```python
from build123d import *

# Parameters (mm, degrees)
SKETCH2_R               = 2.1828125
BOSS_EXTRUDE1_DEPTH     = 3.175
SKETCH3_W               = 36.843225838
SKETCH3_H               = 9.525
BOSS_EXTRUDE2_DEPTH     = 25.4
SKETCH4_R               = 2.1828125
SKETCH4_W               = 0.959112919
SKETCH4_H               = 25.4
SKETCH4_W_2             = 15.875
SKETCH4_H_2             = 15.875
CUT_EXTRUDE1_DEPTH      = 1
CUT_EXTRUDE1_DEPTH_BACK = 10.525
FILLET1_R               = 1.5875
CHAMFER1_SIZE           = 0.396875


with BuildPart() as part:
    # Sketch2 → Boss-Extrude1 (new body)
    with BuildSketch(Plane(origin=(0, 0, 0), x_dir=(1, 0, 0), z_dir=(0, 1, 0))):
        with BuildLine():
            Line((-38.1, 4.7625), (38.1, 4.7625))
            ThreePointArc((38.1, 4.7625), (42.8625, 0), (38.1, -4.7625))
            Line((38.1, -4.7625), (-38.1, -4.7625))
            ThreePointArc((-38.1, -4.7625), (-42.8625, 0), (-38.1, 4.7625))
        make_face()
        with Locations((-38.1, 0)):
            Circle(SKETCH2_R, mode=Mode.SUBTRACT)
        with Locations((38.1, 0)):
            Circle(SKETCH2_R, mode=Mode.SUBTRACT)
    extrude(amount=BOSS_EXTRUDE1_DEPTH)

    # Sketch3 → Boss-Extrude2 (add)
    with BuildSketch(Plane(origin=(0, 3.175, 0), x_dir=(1, 0, 0), z_dir=(0, 1, 0))):
        Rectangle(SKETCH3_W, SKETCH3_H)
    extrude(amount=BOSS_EXTRUDE2_DEPTH)

    # Sketch4 → Cut-Extrude1 (cut, two sides)
    with BuildSketch(Plane.XY.offset(4.7625)) as cut_extrude1_sk:
        with Locations((-12.7, 23.8125)):
            Circle(SKETCH4_R)
        with Locations((12.7, 23.8125)):
            Circle(SKETCH4_R)
        with Locations((-17.94205646, 15.875)):
            Rectangle(SKETCH4_W, SKETCH4_H)
        with Locations((17.94205646, 15.875)):
            Rectangle(SKETCH4_W, SKETCH4_H)
        with Locations((0, 11.1125)):
            Rectangle(SKETCH4_W_2, SKETCH4_H_2)
    extrude(amount=CUT_EXTRUDE1_DEPTH, mode=Mode.SUBTRACT)
    extrude(cut_extrude1_sk.sketch, amount=-CUT_EXTRUDE1_DEPTH_BACK, mode=Mode.SUBTRACT)

    # Fillet1
    fillet1_edges = [part.edges().sort_by_distance(p)[0] for p in [
        (-17.4625, 3.175, 0),
        (-17.4625, 28.575, 0),
        (17.4625, 28.575, 0),
        (17.4625, 3.175, 0),
        (-7.9375, 3.175, 0),
        (-7.9375, 19.05, 0),
        (7.9375, 19.05, 0),
        (7.9375, 3.175, 0),
    ]]
    fillet(fillet1_edges, radius=FILLET1_R)

    # Chamfer1
    chamfer1_edges = [part.edges().sort_by_distance(p)[0] for p in [
        (0, 28.575, -4.7625),
        (0, 28.575, 4.7625),
        (0, 3.175, 4.7625),
        (-7.9375, 11.1125, 4.7625),
        (0, 19.05, 4.7625),
        (7.9375, 11.1125, 4.7625),
        (-17.4625, 15.875, 4.7625),
        (28.575, 3.175, 4.7625),
        (17.4625, 15.875, 4.7625),
        (16.997532015, 28.110032015, 4.7625),
        (-16.997532015, 28.110032015, 4.7625),
        (-17.4625, 15.875, -4.7625),
        (0, 19.05, -4.7625),
        (-7.9375, 11.1125, -4.7625),
        (0, 3.175, -4.7625),
        (7.9375, 11.1125, -4.7625),
        (-28.575, 3.175, -4.7625),
        (17.4625, 15.875, -4.7625),
        (16.997532015, 28.110032015, -4.7625),
        (-16.997532015, 28.110032015, -4.7625),
        (-40.2828125, 0, 0),
        (-17.927467985, 3.639967985, 4.7625),
        (-40.2828125, 3.175, 0),
        (-17.927467985, 3.639967985, -4.7625),
        (17.927467985, 3.639967985, 4.7625),
        (17.927467985, 3.639967985, -4.7625),
        (-7.472532015, 18.585032015, 4.7625),
        (42.8625, 3.175, 0),
        (-7.472532015, 18.585032015, -4.7625),
        (7.472532015, 18.585032015, 4.7625),
        (7.472532015, 18.585032015, -4.7625),
        (7.472532015, 3.639967985, 4.7625),
        (7.472532015, 3.639967985, -4.7625),
        (-7.472532015, 3.639967985, 4.7625),
        (-7.472532015, 3.639967985, -4.7625),
        (35.9171875, 0, 0),
        (35.9171875, 3.175, 0),
        (28.575, 3.175, -4.7625),
        (10.5171875, 23.8125, -4.7625),
        (10.5171875, 23.8125, 4.7625),
        (-42.8625, 3.175, 0),
        (0, 0, -4.7625),
        (42.8625, 0, 0),
        (0, 0, 4.7625),
        (-42.8625, 0, 0),
        (-14.8828125, 23.8125, -4.7625),
        (-14.8828125, 23.8125, 4.7625),
        (-28.575, 3.175, 4.7625),
    ]]
    chamfer(chamfer1_edges, length=CHAMFER1_SIZE)


solid = part.part
```
Build history of the part. All positions in model axes, mm. A direction names the side the tool comes from. Give positions to 0.01 mm unless a question says otherwise; leave off trailing zeros. Loops run counter-clockwise (first coordinate to the right, second up) from the corner with the lowest first, then second, coordinate; pieces in that order, holes last. Notation, with made-up numbers: (-36, 89) -> (-31, 89) arc R24 ccw to (-31, 110) -> close; hole circle Ø7 at (-34, -36). An arc over 180 degrees is marked (long way). One line per question, with ' | ' between items.
Q1. Drill centre lines: line 1 along X through (y, z) = (1.1, 0); line 2 along Y through (x, z) = (0, -2.5) (3 decimals); line 3 along Y through (x, z) = (12.7, -1.25) (3 decimals). Where is each one in solid material? Low to high. Write a range as [from, to].
Filled sheet:
line 1: x = [-42.86, -40.28], [-35.92, 35.92], [40.28, 42.86] | line 2: y = [0, 3.175], [19.05, 28.575] | line 3: y = [0, 21.63], [25.995, 28.575]
Q2. Pull direction Y, two halves, no side cores. Call faces 1 (the conical face through (16.787, 27.919, -4.649)), 2 (the cylindrical face through (-42.86, 1.57, 0.1)), 3 (the cylindrical face through (10.97, 22.48, 0.06)): pulls with the +Y half, pulls with the -Y half, needs draft (parallel to the pull), parting line crosses it, or undercut.
Filled sheet:
face 1: pulls with the +Y half | face 2: needs draft | face 3: undercut
Q3. Cut at B-B, the plane y = 9. Write the cut outline in (x, z), plus the area to 3 significant figures.
Filled sheet:
outline: (-17.46, -4.37) -> (-17.07, -4.76) -> (-8.33, -4.76) -> (-7.94, -4.37) -> (-7.94, 4.37) -> (-8.33, 4.76) -> (-17.07, 4.76) -> (-17.46, 4.37) -> close; (7.94, -4.37) -> (8.33, -4.76) -> (17.07, -4.76) -> (17.46, -4.37) -> (17.46, 4.37) -> (17.07, 4.76) -> (8.33, 4.76) -> (7.94, 4.37) -> close | area: 181 mm²
Q4. Drop flat-ended pins along their axis: pin 1 (4.5 mm diameter, centred on x = 28.5, z = 0, fed in from +Y) (3 decimals); pin 2 (4 mm diameter, centred on y = 10, z = 2.5, fed in from +X); pin 3 (4 mm diameter, centred on y = 24, z = 3.5, fed in from -X). Give the stop position or say it passes through.
Filled sheet:
pin 1: stops at y = 3.175 | pin 2: stops at x = 17.46 | pin 3: stops at x = -17.46
Q5. Cut at D-D, the plane y = 20.5. Write the cut outline in (x, z), plus the area to 3 significant figures.
Filled sheet:
outline: (-17.46, -4.37) -> (-17.07, -4.76) -> (17.07, -4.76) -> (17.46, -4.37) -> (17.46, 4.37) -> (17.07, 4.76) -> (-17.07, 4.76) -> (-17.46, 4.37) -> close | area: 332 mm²
Q6. Cut at C-C, the plane x = -30.5. Write the cut outline in (y, z) (1 decimal), plus the area to 3 significant figures.
Filled sheet:
outline: (0, -4.4) -> (0.4, -4.8) -> (2.8, -4.8) -> (3.2, -4.4) -> (3.2, 4.4) -> (2.8, 4.8) -> (0.4, 4.8) -> (0, 4.4) -> close | area: 29.9 mm²
Q7. Tool access for faces 4 (the flat face through (31, 3.175, 0)), 5 (the cylindrical face through (7.485, 18.573, -0.061)), 6 (the flat face through (-1, 20, -4.762)), 7 (the flat face through (-17.463, 16, 0)): list every direction of +Z, -Z, +X, -X, +Y, -Y with a clear straight run to the whole face (end or side of a thin tool).
Filled sheet:
face 4: +Z, -Z, +X, +Y | face 5: +Z, -Z | face 6: -Z, +X, -X, +Y, -Y | face 7: +Z, -Z, -X, +Y
